```python
from build123d import *

# Parameters (mm, degrees)
F0_W          = 40
F0_H          = 40
F1_DEPTH      = 800
F1_DEPTH_BACK = 800
F4_W          = 40
F4_H          = 100
F5_DEPTH      = 10
F6_W          = 40
F6_H          = 100
F7_DEPTH      = 1
F8_W          = 40
F8_H          = 10
F9_DEPTH      = 800
F9_DEPTH_BACK = 800
F10_W         = 100
F10_H         = 40
F11_DEPTH     = 10
F12_W         = 100
F12_H         = 40
F13_DEPTH     = 10
F14_W         = 50
F14_H         = 120
F14_R         = 7
F15_DEPTH     = 10
F16_W         = 50
F16_H         = 120
F16_R         = 7
F17_DEPTH     = 10


with BuildPart() as f1:
    # F0 (on Right) → F1 (new body, two sides)
    with BuildSketch(Plane.YZ) as f1_sk:
        Rectangle(F0_W, F0_H)
    extrude(amount=F1_DEPTH)
    extrude(f1_sk.sketch, amount=-F1_DEPTH_BACK)

    # F4 (on offset) → F5 (join)
    with BuildSketch(Plane.YZ.offset(-750)):
        with Locations((0, -70)):
            Rectangle(F4_W, F4_H)
    extrude(amount=F5_DEPTH)

    # F6 (on offset) → F7 (join)
    with BuildSketch(Plane.YZ.offset(750)):
        with Locations((0, -70)):
            Rectangle(F6_W, F6_H)
    extrude(amount=-F7_DEPTH)

    # F8 (on Right) → F9 (join, two sides)
    with BuildSketch(Plane.YZ) as f9_sk:
        with Locations((0, -125)):
            Rectangle(F8_W, F8_H)
    extrude(amount=F9_DEPTH)
    extrude(f9_sk.sketch, amount=-F9_DEPTH_BACK)

    # F10 (on face) → F11 (join)
    with BuildSketch(Plane.YZ.offset(800)):
        with Locations((30, -125)):
            Rectangle(F10_W, F10_H)
    extrude(amount=F11_DEPTH)

    # F12 (on face) → F13 (join)
    with BuildSketch(Plane(origin=(-800, 0, 0), x_dir=(0, -1, 0), z_dir=(-1, 0, 0))):
        with Locations((-30, -125)):
            Rectangle(F12_W, F12_H)
    extrude(amount=F13_DEPTH)

    # F14 (on face) → F15 (join)
    with BuildSketch(Plane(origin=(0, 80, 0), x_dir=(-1, 0, 0), z_dir=(0, 1, 0))):
        with Locations((-805, -125)):
            Rectangle(F14_W, F14_H)
        with Locations((-805, -165)):
            Circle(F14_R, mode=Mode.SUBTRACT)
        with Locations((-805, -85)):
            Circle(F14_R, mode=Mode.SUBTRACT)
    extrude(amount=F15_DEPTH)

    # F16 (on face) → F17 (join)
    with BuildSketch(Plane(origin=(0, 80, 0), x_dir=(-1, 0, 0), z_dir=(0, 1, 0))):
        with Locations((805, -125)):
            Rectangle(F16_W, F16_H)
        with Locations((805, -165)):
            Circle(F16_R, mode=Mode.SUBTRACT)
        with Locations((805, -85)):
            Circle(F16_R, mode=Mode.SUBTRACT)
    extrude(amount=F17_DEPTH)


solid = f1.part
```
Verification items for the finished model (mm, model axes). A direction names the side the tool comes from. Give positions to 0.01 mm unless a question says otherwise; leave off trailing zeros. Loops run counter-clockwise (first coordinate to the right, second up) from the corner with the lowest first, then second, coordinate; pieces in that order, holes last.
1. Section check B-B, the plane x = -365.5. Enter the section's corners in (y, z), then the cut area to 3 significant figures.
2. Section check A-A, the plane y = 57. Enter the section's corners in (x, z), then the cut area to 3 significant figures.
3. Set-up check for faces 1 (the flat face through (749, 0, -69)), 2 (the flat face through (775, 0, -20)), 3 (the flat face through (775, 0, -120)): record each of +Z, -Z, +X, -X, +Y, -Y from which the full face is reachable in a straight line by a thin tool's end or side.
4. Mould release check, pull along Y, two halves, no side actions. Record for faces 4 (the flat face through (800, 29, -125)), 5 (the flat face through (-810, 31, -125)), 6 (the flat face through (-800, 31, -125)), 7 (the flat face through (-805, 90, -124)): released by +Y, released by -Y, zero draft, split by the parting line, or undercut.
5. Thickness scan on line 1 (Z direction, x = -805, y = 86); line 2 (X direction, y = -15, z = -111.5); line 3 (X direction, y = 37, z = -123.5). Record the ranges inside material, lowest first.
6. Go/stop test with flat-tipped pins: pin 1 Ø8.5 at (x, z) = (805, -165) entering from -Y; pin 2 Ø20 at (y, z) = (23.5, -130) entering from -X; pin 3 Ø5 at (x, y) = (802.5, 44.5) entering from +Z; pin 4 Ø5 at (y, z) = (1, -21.5) entering from -X. Record where each tip stops, or that it passes through.
Geometry says:
1. outline: (-20, -130) - (20, -130) - (20, -120) - (-20, -120) - close; (-20, -20) - (20, -20) - (20, 20) - (-20, 20) - close
1. area: 2,000 mm2
2. outline: (-810, -145) - (-800, -145) - (-800, -105) - (-810, -105) - close; (800, -145) - (810, -145) - (810, -105) - (800, -105) - close
2. area: 800 mm2
3. face 1: +Y, -Y
3. face 2: +X, +Y, -Y
3. face 3: -Y
4. face 4: undercut
4. face 5: zero draft
4. face 6: undercut
4. face 7: released by +Y
5. line 1: z = -185 to -172, -158 to -92, -78 to -65
5. line 2: x = -810 to -800, -750 to -740, 749 to 750, 800 to 810
5. line 3: x = -810 to -800, 800 to 810
6. pin 1: passes through
6. pin 2: stops at x = -810
6. pin 3: stops at z = -105
6. pin 4: stops at x = -800
